Here's the drawing with two shaded views (mm, measured from the low corner). I have some questions. A direction names the side the tool comes from. Coordinates: 2 decimals unless noted, no trailing zeros. Write each loop counter-clockwise with the first axis right and the second up, starting at its lowest first coordinate (ties: lowest second). Pieces come first, ordered by that corner, then holes.
Item 1: I want a section at C-C on y = 39. Please give me the cut outline in (x, z).
Item 2: I want a section at A-A on z = 3.6. Please give me the cut outline in (x, y) (1 decimal), then the cut area to 3 significant figures.
Item 3: Which directions (+Z, -Z, +X, -X, +Y, -Y) give clear straight access to the entire face, cutting with the end or side of a thin tool? Please do the marked faces 1 and 2.
Item 4: Thinking about a two-plate mould opening in X: for the marked faces 3, 4, 5 and 6, which applies, +X half, -X half, draft (parallel to the pull), parting line (faces both ways), or undercut?
Item 5: For P1, Ø3.5, axis at x = 12, y = 23.5, coming from the +Z side, with a flat end and sliding along its axis, tell me the tip position at first contact or that it passes through.
Item 6: If I drill on probe 1 along Y at (x, z) = (9, 4.25); probe 2 along X at (y, z) = (14.5, 5.05); probe 3 along Y at (x, z) = (7.5, 3.25), over which ranges is the centre line in solid material (lowest first)?
Item 7: I want a section at D-D on x = 6.5. Please give me the cut outline in (y, z).
Item 8: I want a section at B-B on z = 0.65. Please give me the cut outline in (x, y) (1 decimal).
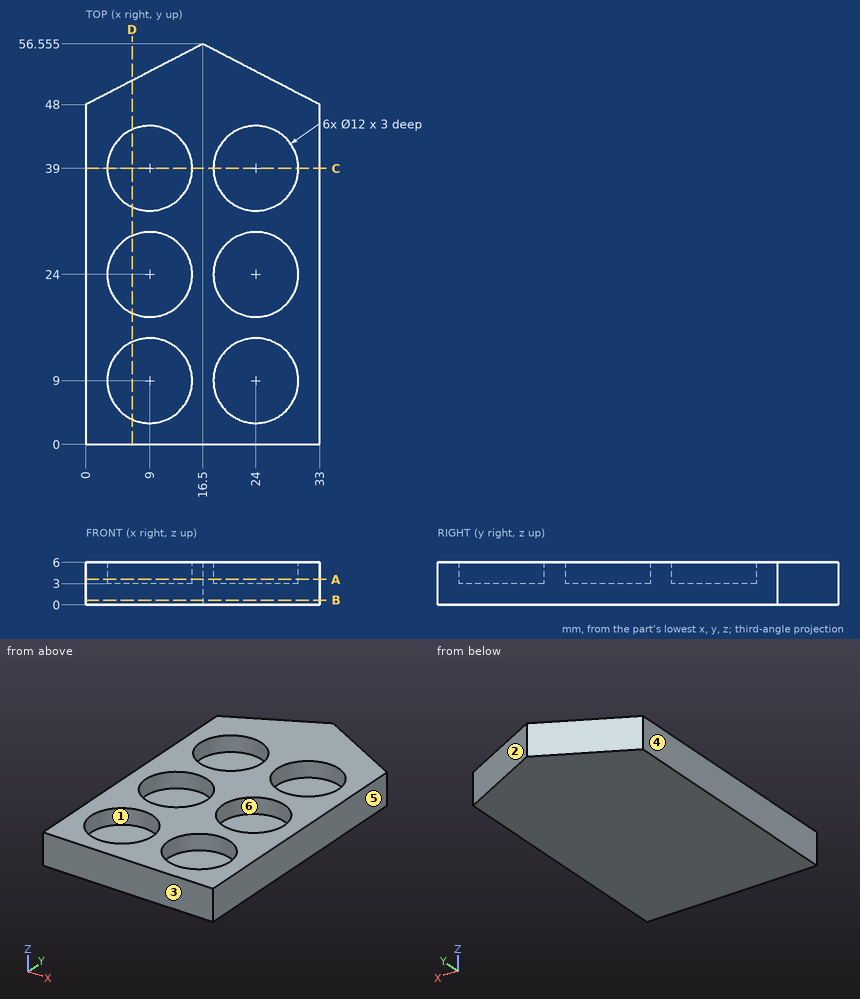
Response values:
1. outline: (0, 0) - (33, 0) - (33, 6) - (30, 6) - (30, 3) - (18, 3) - (18, 6) - (15, 6) - (15, 3) - (3, 3) - (3, 6) - (0, 6) - close
2. outline: (0, 0) - (33, 0) - (33, 48) - (16.5, 56.6) - (0, 48) - close; hole circle Ø12 at (9, 9); hole circle Ø12 at (9, 24); hole circle Ø12 at (9, 39); hole circle Ø12 at (24, 9); hole circle Ø12 at (24, 24); hole circle Ø12 at (24, 39)
2. area: 1,050 mm2
3. face 1: +Z
3. face 2: +Z, -Z, +X, +Y
4. face 3: draft
4. face 4: -X half
4. face 5: +X half
4. face 6: undercut
5. P1: stops at z = 3
6. probe 1: y = 0 to 3, 15 to 18, 30 to 33, 45 to 52.67
6. probe 2: x = 0 to 6.6, 11.4 to 21.6, 26.4 to 33
6. probe 3: y = 0 to 3.19, 14.81 to 18.19, 29.81 to 33.19, 44.81 to 51.89
7. outline: (0, 0) - (51.37, 0) - (51.37, 6) - (44.45, 6) - (44.45, 3) - (33.55, 3) - (33.55, 6) - (29.45, 6) - (29.45, 3) - (18.55, 3) - (18.55, 6) - (14.45, 6) - (14.45, 3) - (3.55, 3) - (3.55, 6) - (0, 6) - close
8. outline: (0, 0) - (33, 0) - (33, 48) - (16.5, 56.6) - (0, 48) - close
